Part model, mm, in its own coordinate system. A direction names the side the tool comes from. Coordinates: 2 decimals unless noted, no trailing zeros. Order: outer loops, then holes, each group sorted by start corner. A loop starts at its lowest first (then second) coordinate and runs counter-clockwise, first axis right, second up.
1) Cut at A-A (y = 5.5). List the corners of the cut face in (x, z), and give its area (3 significant figures).
2) Cut at C-C (z = 116). List the corners of the cut face in (x, y).
3) Tool access for faces 1 (the cylindrical face through (24.5, 24.6, 68.1)), 2 (the flat face through (-27.739, 0, 66)): list every direction of +Z, -Z, +X, -X, +Y, -Y with a clear straight run to the whole face (end or side of a thin tool).
4) Cut at B-B (x = 12). List the corners of the cut face in (y, z).
5) Wall check: L1, parallel to Y at x = -1.5, z = 44; L2, parallel to X at y = 8, z = 17.5; L3, parallel to Y at x = -23.5, z = 118.5. Give the ranges that are in metal, low to high.
```python
from build123d import *

# Parameters (mm, degrees)
F0_W     = 55.477142
F0_H     = 55.65466
F1_DEPTH = 134.265617
F2_R     = 5
F3_T     = -2.5


with BuildPart() as f1:
    # F0 (on Top) → F1 (new body)
    with BuildSketch(Plane.XY):
        Rectangle(F0_W, F0_H)
    extrude(amount=F1_DEPTH)

    # F2
    f2_edges = [f1.edges().sort_by_distance(p)[0] for p in [
        (27.738571, -27.82733, 67.132808),
        (27.738571, 27.82733, 67.132808),
        (-27.738571, -27.82733, 67.132808),
        (-27.738571, 27.82733, 67.132808),
    ]]
    fillet(f2_edges, radius=F2_R)

    # F3
    f3_openings = [f1.faces().sort_by_distance(p)[0] for p in [
        (0, 0, 134.265617),
        (0, 0, 0),
    ]]
    offset(amount=F3_T, openings=f3_openings)


solid = f1.part
```
Geometry check:
1. outline: (-27.74, 0) - (-25.24, 0) - (-25.24, 134.27) - (-27.74, 134.27) - close; (25.24, 0) - (27.74, 0) - (27.74, 134.27) - (25.24, 134.27) - close
1. area: 671 mm2
2. outline: (-27.74, -22.83) arc R5 ccw to (-22.74, -27.83) - (22.74, -27.83) arc R5 ccw to (27.74, -22.83) - (27.74, 22.83) arc R5 ccw to (22.74, 27.83) - (-22.74, 27.83) arc R5 ccw to (-27.74, 22.83) - close; hole (-25.24, -22.83) arc R2.5 ccw to (-22.74, -25.33) - (22.74, -25.33) arc R2.5 ccw to (25.24, -22.83) - (25.24, 22.83) arc R2.5 ccw to (22.74, 25.33) - (-22.74, 25.33) arc R2.5 ccw to (-25.24, 22.83) - close
3. face 1: +Z, -Z
3. face 2: +Z, -Z, -X, +Y, -Y
4. outline: (-27.83, 0) - (-25.33, 0) - (-25.33, 134.27) - (-27.83, 134.27) - close; (25.33, 0) - (27.83, 0) - (27.83, 134.27) - (25.33, 134.27) - close
5. L1: y = -27.83 to -25.33, 25.33 to 27.83
5. L2: x = -27.74 to -25.24, 25.24 to 27.74
5. L3: y = -27.77 to -25.21, 25.21 to 27.77
